Here's how the part is built. I have some questions about the finished solid (model axes, mm). A direction names the side the tool comes from. Round coordinates to 2 decimals unless told otherwise and drop trailing zeros. Order: outer loops, then holes, each group sorted by start corner. A loop starts at its lowest first (then second) coordinate and runs counter-clockwise, first axis right, second up. Notation, with made-up numbers: (52, 56.5) -> (87, 56.5) arc R14 cw to (87, 61.5) -> close; hole circle Ø7 at (70.5, 35.5). An arc over 180 degrees is marked (long way). One line per item, written item: value.
```python
from build123d import *

# Parameters (mm, degrees)
EXTRUDE072_DEPTH = 15
EXTRUDE068_DEPTH = 1
EXTRUDE067_DEPTH = 1


with BuildPart() as extrude072:
    # Sketch269 → Extrude072 (new body)
    with BuildSketch(Plane.YZ):
        with BuildLine():
            ThreePointArc((6, 0), (6.707107, 0.292893), (7, 1))
            Line((7, 1), (7, 0))
            Line((6, 0), (7, 0))
        make_face()
    extrude(amount=EXTRUDE072_DEPTH)


with BuildPart() as extrude068:
    # Sketch265 → Extrude068 (new body)
    with BuildSketch(Plane.XY):
        with BuildLine():
            ThreePointArc((10.5, 1), (11.5, 2), (10.5, 3))
            Line((10.5, 3), (2.5, 3))
            ThreePointArc((2.5, 3), (1.5, 2), (2.5, 1))
            Line((2.5, 1), (10.5, 1))
        make_face()
    extrude(amount=EXTRUDE068_DEPTH)


with BuildPart() as cut043:
    # Sketch264 → Extrude067 (new body)
    with BuildSketch(Plane.XY):
        with BuildLine():
            ThreePointArc((0, 1), (0.292893, 0.292893), (1, 0))
            Line((1, 0), (11, 0))
            ThreePointArc((11, 0), (11.707107, 0.292893), (12, 1))
            Line((12, 4), (12, 1))
            ThreePointArc((13, 5), (12.292893, 4.707107), (12, 4))
            Line((13, 7), (13, 5))
            Line((0, 7), (13, 7))
            Line((0, 1), (0, 7))
        make_face()
    extrude(amount=EXTRUDE067_DEPTH)

    # Cut040: cut Extrude068
    add(extrude068.part, mode=Mode.SUBTRACT)

    # Cut043: cut Extrude072
    add(extrude072.part, mode=Mode.SUBTRACT)


solid = cut043.part
```
Q1. I want a section at A-A on y = 2. Write out the boundary of the cut face in (x, z), then the cut area to 3 significant figures.
Answers:
outline: (0, 0) -> (1.5, 0) -> (1.5, 1) -> (0, 1) -> close; (11.5, 0) -> (12, 0) -> (12, 1) -> (11.5, 1) -> close
area: 2.00 mm2
Q2. I want a section at B-B on x = 6.5. Write out the boundary of the cut face in (y, z).
Answers:
outline: (0, 0) -> (1, 0) -> (1, 1) -> (0, 1) -> close; (3, 0) -> (6, 0) arc R1 ccw to (7, 1) -> (3, 1) -> close
Q3. Which directions (+Z, -Z, +X, -X, +Y, -Y) give clear straight access to the entire face, cutting with the end or side of a thin tool? Please do faces 1 (the face through (5.9, 0, 0.5)), 2 (the face through (12, 2.5, 0.5)), 3 (the face through (6.6, 3, 0.5)).
Answers:
face 1: +Z, -Z, +X, -X, -Y
face 2: +Z, -Z, +X, -Y
face 3: +Z, -Z
Q4. I want a section at D-D on y = 0.5. Write out the boundary of the cut face in (x, z).
Answers:
outline: (0.13, 0) -> (11.87, 0) -> (11.87, 1) -> (0.13, 1) -> close
Q5. If we mould it in two halves opening along X, with no side actions, what happens to faces 4 (the face through (5, 4, 0)), 5 (the face through (13, 6, 0.5)), 6 (the face through (11.5, 2, 0.5))? For each: pulls with the +X half, pulls with the -X half, needs draft (parallel to the pull), parting line crosses it, or undercut.
Answers:
face 4: needs draft
face 5: pulls with the +X half
face 6: undercut
Q6. I want a section at C-C on z = 0.7. Write out the boundary of the cut face in (x, y).
Answers:
outline: (0, 1) arc R1 ccw to (1, 0) -> (11, 0) arc R1 ccw to (12, 1) -> (12, 4) arc R1 cw to (13, 5) -> (13, 6.95) -> (0, 6.95) -> close; hole (2.5, 1) -> (10.5, 1) arc R1 ccw to (10.5, 3) -> (2.5, 3) arc R1 ccw to start
Q7. I need wall thicknesses on line 1 along X through (y, z) = (2, 0.1); line 2 along Y through (x, z) = (8, 0.55); line 3 along Y through (x, z) = (2.5, 0.9). Which ranges of each line are inside material? Lowest first, please.
Answers:
line 1: 0 to 1.5, 11.5 to 12
line 2: 0 to 1, 3 to 6.89
line 3: 0 to 1, 3 to 6.99
